The model under review builds one solid part; all positions refer to its coordinate system, in mm. A direction names the side the tool comes from. Give positions to 0.01 mm unless a question says otherwise; leave off trailing zeros. Order: outer loops, then holes, each group sorted by start corner. A loop starts at its lowest first (then second) coordinate and runs counter-clockwise, first axis right, second up. Notation, with made-up numbers: (-18, 79) - (41, 79) arc R17 ccw to (41, 108) - close; hole circle Ø10 at (33.25, 37.25). An arc over 180 degrees is marked (long way). Use a Markdown table: item, result. Add a question column.
```python
from build123d import *

# Parameters (mm, degrees)
F1_DEPTH = 15
F2_R     = 2.5
F3_DEPTH = 15
F4_R     = 4.5
F4_R_2   = 2.5
F5_DEPTH = 3
F7_DEPTH = 30
F8_R     = 4
F9_DEPTH = 8


with BuildPart() as f1:
    # F0 (on Top) → F1 (new body, symmetric)
    with BuildSketch(Plane.XY):
        with BuildLine():
            ThreePointArc((-15, 0), (0, 15), (15, 0))
            Line((15, 0), (40, 0))
            Line((40, 0), (40, 10))
            Line((40, 10), (22.912878, 10))
            ThreePointArc((22.912878, 10), (0, 25), (-22.912878, 10))
            Line((-22.912878, 10), (-40, 10))
            Line((-40, 10), (-40, 0))
            Line((-40, 0), (-15, 0))
        make_face()
    extrude(amount=F1_DEPTH, both=True)

    # F2 (on face) → F3 (cut)
    with BuildSketch(Plane(origin=(0, 10, 0), x_dir=(-1, 0, 0), z_dir=(0, 1, 0))):
        with Locations((-31.456439, 9)):
            Circle(F2_R)
        with Locations((-31.456439, -9)):
            Circle(F2_R)
        with Locations((31.456439, -9)):
            Circle(F2_R)
        with Locations((31.456439, 9)):
            Circle(F2_R)
    extrude(amount=-F3_DEPTH, mode=Mode.SUBTRACT)

    # F4 (on face) → F5 (cut)
    with BuildSketch(Plane(origin=(0, 10, 0), x_dir=(-1, 0, 0), z_dir=(0, 1, 0))):
        with Locations((31.456439, 9)):
            Circle(F4_R)
        with Locations((31.456439, 9)):
            Circle(F4_R_2, mode=Mode.SUBTRACT)
        with Locations((31.456439, -9)):
            Circle(F4_R)
        with Locations((-31.456439, -9)):
            Circle(F4_R)
        with Locations((-31.456439, 9)):
            Circle(F4_R)
    extrude(amount=-F5_DEPTH, mode=Mode.SUBTRACT)

    # F6 (on face) → F7 (join)
    with BuildSketch(Plane.XY.offset(15)):
        Polygon((-9.797959, 33), (-9.797959, 23), (9.797959, 23), (9.797959, 33), (0, 33), align=None)
        Polygon((-25, 33), (-9.797959, 33), (0, 33), (0, 40), (-25, 40), align=None)
        Polygon((0, 33), (9.797959, 33), (25, 33), (25, 40), (0, 40), align=None)
    extrude(amount=-F7_DEPTH)

    # F8 (on face) → F9 (cut)
    with BuildSketch(Plane(origin=(0, 40, 0), x_dir=(-1, 0, 0), z_dir=(0, 1, 0))):
        with Locations((16, 8)):
            Circle(F8_R)
        with Locations((16, -8)):
            Circle(F8_R)
        with Locations((-16, -8)):
            Circle(F8_R)
        with Locations((-16, 8)):
            Circle(F8_R)
    extrude(amount=-F9_DEPTH, mode=Mode.SUBTRACT)


solid = f1.part
```
Q1. We need section B-B (z = 0.5). Write out the cut boundary in (x, y), plus the area to 3 significant figures.
Q2. We need section C-C (x = -16). Write out the cut boundary in (y, z).
Q3. We need section A-A (y = 9). Write out the cut boundary in (x, z).
Q4. Wall thickness on probe 1 along Z at (x, y) = (16, 35.25); probe 2 along Y at (x, z) = (-24, 11); probe 3 along Y at (x, z) = (32.5, -2.25): over which ranges is each line inside the solid? List them lowest first.
Q5. Clearance check with flat-ended pins moving along their axes: P1, Ø6.5, axis at x = -31.46, z = -9, coming from the +Y side; P2, Ø8, axis at x = 20, y = 22.5, coming from the +Z side; P3, Ø1, axis at y = 16.5, z = -11, coming from the +X side; P4, Ø2, axis at y = 24.5, z = 5.5, coming from the -X side. State where each tip first meets the part, or that it passes through.
Q6. We need section D-D (z = -9). Count the separate pieces of the cut face and the enclosed holes in it, plus the area to 3 significant figures.
Q7. Draft analysis for pull direction Y (two halves, no side actions). For faces 5 (the flat face through (-1, 20, 15)), 6 (the cylindrical face through (17.693, 17.662, 0.21)), 7 (the flat face through (-33.4, 7, 7.1)), state which applies: pulls with the +Y half, pulls with the -Y half, needs draft (parallel to the pull), parting line crosses it, or undercut.
Q8. Machinability: for faces 1 (the flat face through (-18, 33, 0)), 2 (the cylindrical face through (33.44, 3.55, 7.48)), 3 (the flat face through (32, 10, 0)), 4 (the flat face through (29.5, 7, 7.1)), which of the approach directions +Z, -Z, +X, -X, +Y, -Y give a long, thin tool a straight path to every point of the face, cutting with its end or side? Answer none if there is none.
Here are the results:
| question | item | result |
|---|---|---|
| 1 | outline | (-40, 0) - (-15, 0) arc R15 cw to (15, 0) - (40, 0) - (40, 10) - (22.91, 10) arc R25 ccw to (9.8, 23) - (9.8, 33) - (25, 33) - (25, 40) - (-25, 40) - (-25, 33) - (-9.8, 33) - (-9.8, 23) arc R25 ccw to (-22.91, 10) - (-40, 10) - close |
| 1 | area | 1,460 mm2 |
| 2 | outline | (0, -15) - (19.21, -15) - (19.21, 15) - (0, 15) - close; (33, -15) - (40, -15) - (40, -12) - (33, -12) - close; (33, -4) - (40, -4) - (40, 4) - (33, 4) - close; (33, 12) - (40, 12) - (40, 15) - (33, 15) - close |
| 3 | outline | (-40, -15) - (-12, -15) - (-12, 15) - (-40, 15) - close; (12, -15) - (40, -15) - (40, 15) - (12, 15) - close; hole circle Ø9 at (-31.46, -9); hole circle Ø9 at (-31.46, 9); hole circle Ø9 at (31.46, -9); hole circle Ø9 at (31.46, 9) |
| 4 | probe 1 | -15 to -12, -4 to 4, 12 to 15 |
| 4 | probe 2 | 0 to 10, 33 to 40 |
| 4 | probe 3 | 0 to 10 |
| 5 | P1 | y = 7 |
| 5 | P2 | through |
| 5 | P3 | x = 19.21 |
| 5 | P4 | x = -9.8 |
| 6 | separate pieces | 5 |
| 6 | enclosed holes | 0 |
| 6 | area | 1,230 mm2 |
| 7 | face 5 | needs draft |
| 7 | face 6 | undercut |
| 7 | face 7 | pulls with the +Y half |
| 8 | face 1 | +Z, -Z, -X |
| 8 | face 2 | +Y, -Y |
| 8 | face 3 | +Z, -Z, +X |
| 8 | face 4 | +Y |
